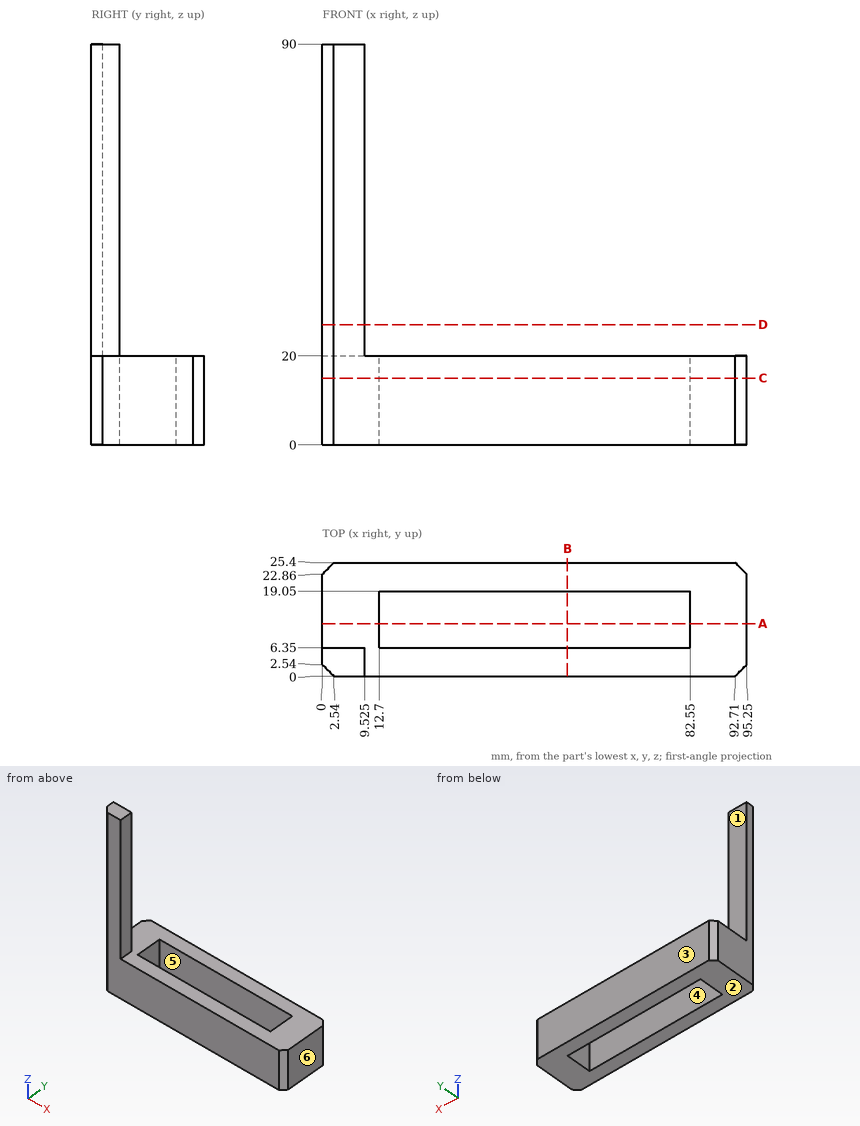
Geometry: see drawing. Coordinates: mm, zero at the bounding-box minimum. A direction names the side the tool comes from. Coordinates: 2 decimals unless noted, no trailing zeros. Order: outer loops, then holes, each group sorted by start corner. A loop starts at its lowest first (then second) coordinate and runs counter-clockwise, first axis right, second up. Notation, with made-up numbers: (18, 38) -> (35, 38) arc R18 ccw to (35, 72) -> close; hole circle Ø6 at (-31.75, -1). An arc over 180 degrees is marked (long way). Write each question's results on one line, items separated by ' | '. Start each with the question number.
1) Cut plane D-D, the plane z = 27. Output: boundary loops of the cut face in (x, y) (3 decimals), and give its area (3 significant figures).
2) Cut plane A-A, the plane y = 11.75. Output: boundary loops of the cut face in (x, z), and give its area (3 significant figures).
3) Set-up query: the marked faces 1 and 2. Return all of +Z, -Z, +X, -X, +Y, -Y with unobstructed straight access to the full face (end or side cutting, diameter ignored); none if empty.
4) Cut plane C-C, the plane z = 15. Output: boundary loops of the cut face in (x, y).
5) First-contact query: pin 1 (1.9 mm diameter, centred on y = 3, z = 70, fed in from +X) (3 decimals); pin 2 (8 mm diameter, centred on x = 78, y = 9, fed in from +Z); pin 3 (5 mm diameter, centred on x = 5.5, z = 62.5, fed in from +Y). Flat tips, straight axial feed; report the tip coordinate or a pass-through.
6) Cut plane B-B, the plane x = 55. Output: boundary loops of the cut face in (y, z), and give its area (3 significant figures).
7) Material intervals for line 1 along Y through (x, z) = (74.5, 10); line 2 along X through (y, z) = (16.75, 4); line 3 along Z through (x, y) = (69, 3.5), sorted ascending.
8) Mould query, pull axis X, two halves, no side actions, for the marked faces 3, 4, 5 and 6. Classes: released by +X, released by -X, zero draft, split by the parting line, or undercut.
Checks:
1) outline: (0, 2.54) -> (2.54, 0) -> (9.525, 0) -> (9.525, 6.35) -> (0, 6.35) -> close | area: 57.3 mm^2
2) outline: (0, 0) -> (12.7, 0) -> (12.7, 20) -> (0, 20) -> close; (82.55, 0) -> (95.25, 0) -> (95.25, 20) -> (82.55, 20) -> close | area: 508 mm^2
3) face 1: +Z, +X, -X, +Y | face 2: -Z, +X, -X, +Y, -Y
4) outline: (0, 2.54) -> (2.54, 0) -> (92.71, 0) -> (95.25, 2.54) -> (95.25, 22.86) -> (92.71, 25.4) -> (2.54, 25.4) -> (0, 22.86) -> close; hole (12.7, 6.35) -> (82.55, 6.35) -> (82.55, 19.05) -> (12.7, 19.05) -> close
5) pin 1: x = 9.525 | pin 2: z = 20 | pin 3: y = 6.35
6) outline: (0, 0) -> (6.35, 0) -> (6.35, 20) -> (0, 20) -> close; (19.05, 0) -> (25.4, 0) -> (25.4, 20) -> (19.05, 20) -> close | area: 254 mm^2
7) line 1: 0 to 6.35, 19.05 to 25.4 | line 2: 0 to 12.7, 82.55 to 95.25 | line 3: 0 to 20
8) face 3: zero draft | face 4: undercut | face 5: undercut | face 6: released by +X
